from build123d import *

# Parameters (mm, degrees)
SKETCH1_W           = 40
SKETCH1_H           = 28
BOSS_EXTRUDE1_DEPTH = 10
SKETCH2_R           = 2.5
BOSS_EXTRUDE2_DEPTH = 9
LPATTERN1_COUNT     = 2
LPATTERN1_PITCH     = 21
FILLET1_R           = 6


with BuildPart() as part:
    # Sketch1 → Boss-Extrude1 (new body)
    with BuildSketch(Plane(origin=(0, 0, 0), x_dir=(0, 0, -1), z_dir=(1, 0, 0))):
        Rectangle(SKETCH1_W, SKETCH1_H)
    extrude(amount=BOSS_EXTRUDE1_DEPTH)

    # Sketch2 → Boss-Extrude2 (add)
    with BuildSketch(Plane.XY.offset(20)):
        with BuildLine():
            Line((10, 19.05), (10, -19.05))
            ThreePointArc((10, -19.05), (5, -24.05), (0, -19.05))
            Line((0, -19.05), (0, 19.05))
            ThreePointArc((0, 19.05), (5, 24.05), (10, 19.05))
        make_face()
        with Locations((5, 19.05)):
            Circle(SKETCH2_R, mode=Mode.SUBTRACT)
        with Locations((5, -19.05)):
            Circle(SKETCH2_R, mode=Mode.SUBTRACT)
    boss_extrude2 = extrude(amount=-BOSS_EXTRUDE2_DEPTH)

    # LPattern1: Boss-Extrude2 ×2
    with Locations(*[(0, 0, -i * LPATTERN1_PITCH) for i in range(1, LPATTERN1_COUNT)]):
        add(boss_extrude2)

    # Fillet1
    fillet1_edges = [part.edges().sort_by_distance(p)[0] for p in [
        (10, -14, 5),
        (0, 14, 5),
        (10, -14, -15),
        (0, 14, -15),
    ]]
    fillet(fillet1_edges, radius=FILLET1_R)


solid = part.part
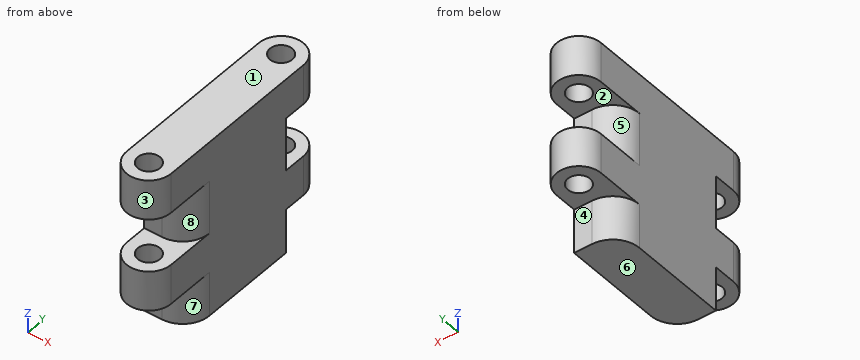
Input: part model. Units: mm. Frame: model coordinates. Face numbers are marked on the shaded views. A direction names the side the tool comes from. Coordinates: 2 decimals unless noted, no trailing zeros. Loops run counter-clockwise (first coordinate to the right, second up) from the corner with the lowest first, then second, coordinate; pieces in that order, holes last. Notation, with made-up numbers: (20.25, -1) -> (51.25, -1) arc R27 ccw to (51.25, 33) -> close; hole circle Ø11 at (15, 9.25). An arc over 180 degrees is marked (long way). Write each question's results on one line, items separated by ' | '. Start each with the question number.
Q1. Section B-B, the plane z = -2.5. Return the cut outline in (x, y), plus the area to 3 significant figures.
Q2. Ray query, line 1 (Y direction, x = 5, z = 17.75); line 2 (X direction, y = -19, z = -3); line 3 (Y direction, x = 6, z = 14). Return the intervals inside material, ascending. Write a range as from..to.
Q3. Section C-C, the plane x = 5. State how many separate pieces and enclosed holes the cut face has, plus the area to 3 significant figures.
Q4. Section D-D, the plane y = -13. Return the cut outline in (x, z), plus the area to 3 significant figures.
Q5. Reachability of the marked faces 4, 5, 6, 7 and 8 from +Z, -Z, +X, -X, +Y, -Y: full face, straight path, thin tool, end or side. Return the list, or none.
Q6. Pull-direction query (Z, two-part tool) for the marked faces 1, 2 and 3; classes: released by +Z, released by -Z, zero draft, split by the parting line, or undercut.
Q7. Pin query (flat end, axial travel): pin 1 (2 mm diameter, centred on x = 7.5, z = -9.5, fed in from -Y); pin 2 (2 mm diameter, centred on x = 1, z = -15, fed in from -Y); pin 3 (5 mm diameter, centred on x = 2.5, y = 16, fed in from -Z). Return the tip coordinate at first contact, or that it passes through.
Q8. Section A-A, the plane y = -20. Return the cut outline in (x, z), plus the area to 3 significant figures.
Found:
1) outline: (0, -19.05) arc R5 ccw to (10, -19.05) -> (10, 19.05) arc R5 ccw to (0, 19.05) -> close; hole circle Ø5 at (5, -19.05); hole circle Ø5 at (5, 19.05) | area: 420 mm2
2) line 1: -24.05..-21.55, -16.55..16.55, 21.55..24.05 | line 2: 0..2.5, 7.5..10 | line 3: -23.95..-21.34, -16.76..16.76, 21.34..23.95
3) separate pieces: 5 | enclosed holes: 0 | area: 1,300 mm2
4) outline: (0, -20) -> (7.32, -20) -> (7.32, -10) -> (10, -10) -> (10, -1) -> (7.32, -1) -> (7.32, 11) -> (10, 11) -> (10, 20) -> (0, 20) -> close | area: 341 mm2
5) face 4: -Z, +X, -X, +Y | face 5: -X, +Y | face 6: -Z, +X, -X, +Y, -Y | face 7: -Z, +X, -Y | face 8: +X, -Y
6) face 1: released by +Z | face 2: undercut | face 3: zero draft
7) pin 1: y = -23.82 | pin 2: y = -14 | pin 3: z = -10
8) outline: (0.09, -10) -> (2.69, -10) -> (2.69, -1) -> (0.09, -1) -> close; (0.09, 11) -> (2.69, 11) -> (2.69, 20) -> (0.09, 20) -> close; (7.31, -10) -> (9.91, -10) -> (9.91, -1) -> (7.31, -1) -> close; (7.31, 11) -> (9.91, 11) -> (9.91, 20) -> (7.31, 20) -> close | area: 93.5 mm2
